Design review of the part built by this model. Coordinates are the model's own, in mm. A direction names the side the tool comes from. Coordinates: 2 decimals unless noted, no trailing zeros. Order: outer loops, then holes, each group sorted by start corner. A loop starts at its lowest first (then second) coordinate and runs counter-clockwise, first axis right, second up. Notation, with made-up numbers: (54, 50) -> (67, 50) arc R27 ccw to (67, 75) -> close; hole circle Ø5 at (34, 76.5). An arc over 180 degrees is marked (long way). Use a Markdown table: item, result. Add a question column.
Q1. Wall thickness on probe 1 along Y at (x, z) = (0, 34); probe 2 along X at (y, z) = (4.5, 0); probe 3 along X at (y, z) = (78.5, 32.5): over which ranges is each line inside the solid? List them lowest first.
Q2. Add section A-A (y = 71). State the section outline as (x, z) points.
Q3. Add section B-B (z = 0). State the section outline as (x, y) points.
Q4. Add section C-C (x = 0). State the section outline as (y, z) points.
Q5. Insertion check: pin 1 (15 mm diameter, centred on x = -3.5, z = 5.5, fed in from -Y). The pin has a flat end and moves straight along its axis. Give the tip position at first contact, or say it passes through.
Q6. Add section D-D (z = 30.5). State the section outline as (x, y) points.
Q7. Machinability: for faces 1 (the face through (-3.252, 56.357, 31.32)), 2 (the face through (0, 10, 0)), 3 (the face through (-32, 51, 1)), which of the approach directions +Z, -Z, +X, -X, +Y, -Y give a long, thin tool a straight path to every point of the face, cutting with its end or side? Answer none if there is none.
Q8. The part is to be moulded in two halves that separate along X. For faces 4 (the face through (0, 51, 36.25)), 5 (the face through (32, 51, 1)), 6 (the face through (0, 71, 26.25)), say which applies: pulls with the +X half, pulls with the -X half, needs draft (parallel to the pull), parting line crosses it, or undercut.
from build123d import *

# Parameters (mm, degrees)
SKETCH1_W           = 64
SKETCH1_H           = 72.5
BOSS_EXTRUDE1_DEPTH = 103
SKETCH2_R           = 15
CUT_EXTRUDE1_DEPTH  = 10
SKETCH3_R           = 15
CUT_EXTRUDE2_DEPTH  = 10


with BuildPart() as part:
    # Sketch1 → Boss-Extrude1 (new body)
    with BuildSketch(Plane(origin=(0, 0, 0), x_dir=(1, 0, 0), z_dir=(0, 1, 0))):
        Rectangle(SKETCH1_W, SKETCH1_H)
    extrude(amount=BOSS_EXTRUDE1_DEPTH)

    # Sketch2 → Cut-Extrude1 (cut)
    with BuildSketch(Plane.XY.offset(36.25)):
        with Locations((0, 71)):
            Circle(SKETCH2_R)
    extrude(amount=-CUT_EXTRUDE1_DEPTH, mode=Mode.SUBTRACT)

    # Sketch3 → Cut-Extrude2 (cut)
    with BuildSketch(Plane.XZ):
        with Locations(Location((0, 0, 0), (0, 0, 270))):
            Circle(SKETCH3_R)
    extrude(amount=-CUT_EXTRUDE2_DEPTH, mode=Mode.SUBTRACT)


solid = part.part
Established:
| question | item | result |
|---|---|---|
| 1 | probe 1 | 0 to 56, 86 to 103 |
| 1 | probe 2 | -32 to -15, 15 to 32 |
| 1 | probe 3 | -32 to -12.99, 12.99 to 32 |
| 2 | outline | (-32, -36.25) -> (32, -36.25) -> (32, 36.25) -> (15, 36.25) -> (15, 26.25) -> (-15, 26.25) -> (-15, 36.25) -> (-32, 36.25) -> close |
| 3 | outline | (-32, 0) -> (-15, 0) -> (-15, 10) -> (15, 10) -> (15, 0) -> (32, 0) -> (32, 103) -> (-32, 103) -> close |
| 4 | outline | (0, -36.25) -> (103, -36.25) -> (103, 36.25) -> (86, 36.25) -> (86, 26.25) -> (56, 26.25) -> (56, 36.25) -> (0, 36.25) -> (0, 15) -> (10, 15) -> (10, -15) -> (0, -15) -> close |
| 5 | pin 1 | y = 10 |
| 6 | outline | (-32, 0) -> (32, 0) -> (32, 103) -> (-32, 103) -> close; hole circle Ø30 at (0, 71) |
| 7 | face 1 | +Z |
| 7 | face 2 | -Y |
| 7 | face 3 | +Z, -Z, -X, +Y, -Y |
| 8 | face 4 | needs draft |
| 8 | face 5 | pulls with the +X half |
| 8 | face 6 | undercut |
